Geometry: final body of the model. Coordinates: model frame, mm. A direction names the side the tool comes from. Round coordinates to 2 decimals unless told otherwise and drop trailing zeros. Loops run counter-clockwise (first coordinate to the right, second up) from the corner with the lowest first, then second, coordinate; pieces in that order, holes last. Notation, with made-up numbers: (21, 66) - (69, 66) arc R19 ccw to (69, 97) - close; hole circle Ø9 at (31, -20). An arc over 180 degrees is marked (long way). Return JSON: item names as keys, results as strings. Group by question number.
1. Section B-B on x = -15.5. Return loops of the section in (y, z), and give its area (3 significant figures).
2. Draft query along X for faces 1 (the face through (-42, 6, 20)), 2 (the face through (36.5, 3, 23.9)), 3 (the face through (51.556, -10, 0)). Return one class per face: +X half, -X half, draft (parallel to the pull), parting line (faces both ways), or undercut.
3. Section C-C on z = -9. Return loops of the section in (x, y), and give its area (3 significant figures).
4. First-contact query: pin 1 Ø8 at (x, z) = (24, 9) entering from -Y; pin 2 Ø10 at (x, z) = (4.5, 21) entering from -Y; pin 3 Ø1 at (x, z) = (-8.5, 6.5) entering from +Y. Flat tips, straight axial feed; report the tip coordinate or a pass-through.
5. Section D-D on y = 3.25. Return loops of the section in (x, z).
6. Set-up query: faces 4 (the face through (-1, -12, 25.177)), 5 (the face through (-1, -10, 29.177)), 6 (the face through (34.963, 2.958, -18.488)). Return all of +Z, -Z, +X, -X, +Y, -Y with unobstructed straight access to the full face (end or side cutting, diameter ignored); none if empty.
7. Section A-A on y = -12.25. Return loops of the section in (x, z), and give its area (3 significant figures).
8. Material intervals for probe 1 along X at (y, z) = (-15, 24); probe 2 along Z at (x, y) = (-42, 2.75); probe 3 along Z at (x, y) = (-10.5, -17.25), sorted ascending.
from build123d import *

# Parameters (mm, degrees)
F0_W     = 103.111512
F0_H     = 58.354322
F1_DEPTH = 20
F2_T     = -4
F3_R     = 6
F4_DEPTH = 6


with BuildPart() as f1:
    # F0 (on Front) → F1 (new body)
    with BuildSketch(Plane.XZ):
        Rectangle(F0_W, F0_H)
    extrude(amount=F1_DEPTH)

    # F2
    f2_openings = [f1.faces().sort_by_distance(p)[0] for p in [
        (0, -20, 0),
    ]]
    offset(amount=F2_T, openings=f2_openings)

    # F3 (on Front) → F4 (join)
    with BuildSketch(Plane.XZ):
        with Locations((-42.373065, -18.751857)):
            Circle(F3_R)
        with Locations((40.957681, -18.751857)):
            Circle(F3_R)
        with Locations((40.957681, 19.885929)):
            Circle(F3_R)
        with Locations((-42.373065, 19.885929)):
            Circle(F3_R)
    extrude(amount=-F4_DEPTH)


solid = f1.part
Taken from the geometry:
{
 "1": {"outline": "(-20, -29.18) - (0, -29.18) - (0, 29.18) - (-20, 29.18) - (-20, 25.18) - (-4, 25.18) - (-4, -25.18) - (-20, -25.18) - close", "area": "361 mm2"},
 "2": {"face 1": "draft", "face 2": "undercut", "face 3": "+X half"},
 "3": {"outline": "(-51.56, -20) - (-47.56, -20) - (-47.56, -4) - (47.56, -4) - (47.56, -20) - (51.56, -20) - (51.56, 0) - (-51.56, 0) - close", "area": "540 mm2"},
 "4": {"pin 1": "y = -4", "pin 2": "y = -20", "pin 3": "y = 0"},
 "5": {"outline": "circle Ø12 at (-42.37, -18.75); circle Ø12 at (-42.37, 19.89); circle Ø12 at (40.96, -18.75); circle Ø12 at (40.96, 19.89)"},
 "6": {"face 4": "-Y", "face 5": "+Z, +X, -X, +Y, -Y", "face 6": "+Y"},
 "7": {"outline": "(-51.56, -29.18) - (51.56, -29.18) - (51.56, 29.18) - (-51.56, 29.18) - close; hole (-47.56, -25.18) - (47.56, -25.18) - (47.56, 25.18) - (-47.56, 25.18) - close", "area": "1,230 mm2"},
 "8": {"probe 1": "-51.56 to -47.56, 47.56 to 51.56", "probe 2": "-24.74 to -12.76, 13.9 to 25.87", "probe 3": "-29.18 to -25.18, 25.18 to 29.18"}
}
